Source: CAD feature listing. Evaluate the final solid. Frame: model axes, mm. A direction names the side the tool comes from. Round coordinates to 2 decimals unless told otherwise and drop trailing zeros. Loops run counter-clockwise (first coordinate to the right, second up) from the corner with the lowest first, then second, coordinate; pieces in that order, holes last.
Item 1: Pull-direction query (Y, two-part tool) for faces 1 (the cylindrical face through (266.488, 40.887, 7.465)), 2 (the flat face through (152, 25, 5)), 3 (the flat face through (161, 41, 10)); classes: released by +Y, released by -Y, zero draft, split by the parting line, or undercut.
Item 2: Section query B-B on z = 3. Return loops of the section in (x, y).
Item 3: Section query C-C on x = 206. Return loops of the section in (y, z).
Item 4: Ray query, L1, parallel to X at y = 21, z = 4; L2, parallel to Z at x = 240, y = 83; L3, parallel to Y at x = 168, z = 1. Return the intervals inside material, ascending.
Item 5: Section query D-D on x = 98.5. Return loops of the section in (y, z), then the cut area to 3 significant figures.
Item 6: Section query A-A on x = 174.5. Return loops of the section in (y, z), then the cut area to 3 significant figures.
Item 7: Access query for faces 4 (the flat face through (151, 20, 5)), 5 (the flat face through (269, 44, 2)), 6 (the flat face through (119.3, 64.4, 7.5)), 7 (the cylindrical face through (1.2, 39.8, 7.5)), 8 (the flat face through (119.291, 15.596, 7.465)). Directions: +Z, -Z, +X, -X, +Y, -Y. A direction counts if a zero-diameter tool reaches every point of the face in a straight line with its end or side. Return the directions, or none.
Item 8: First-contact query: P1, Ø2.5, axis at y = 21.5, z = 4.5, coming from the -X side; P2, Ø1, axis at y = 34.5, z = 8.5, coming from the -X side; P3, Ø5, axis at x = 160.5, z = 6, coming from the +Y side. Flat tips, straight axial feed; report the tip coordinate or a pass-through.
Autodesk Inventor part; units mm, degrees
ref_plane "YZ Plane" through (0, 0, 0) normal (1, 0, 0) x (0, 1, 0)
ref_plane "XZ Plane" through (0, 0, 0) normal (0, 1, 0) x (-1, 0, 0)
ref_plane "XY Plane" through (0, 0, 0) normal (0, 0, 1) x (1, 0, 0)
sketch "Boceto1" plane through (0, 0, 0) normal (0, 0, 1) x (1, 0, 0)
  circle A0 centre (229, 39.9983) radius 35 construction
  line L0 (269, 87.6892) -> (269, -0.002)
  line L1 (269, -0.002) -> (0, 0)
  line L2 (0, 0) -> (0, 54.8968)
  line L3 (457.9938, -0.0034) -> (457.9938, 80) construction
  line L4 (457.9938, 80) -> (-432.9938, 80) construction
  line L5 (189, -0.0014) -> (189, 79.998) construction
  line L6 (189, 79.998) -> (269, 79.998) construction
  circle A1 centre (229, 39.9983) radius 11.3 construction
  line L7 (119, 54.9966) -> (199, 54.9966) construction
  line L8 (199, 54.9966) -> (199, 25) construction
  line L9 (199, 25) -> (119, 25) construction
  line L10 (119, 25) -> (119, 54.9966) construction
  arc A2 (224.4624, 2.7754) -> (224.4624, 77.2212) centre (229, 39.9983) ccw
  arc A3 (11.1326, 51.2153) -> (11.1326, 28.7814) centre (12.5, 39.9983) ccw
  line L11 (224.4624, 77.2212) -> (11.1326, 51.2153)
  line L12 (224.4624, 2.7754) -> (11.1326, 28.7814)
  line L13 (0, 54.8968) -> (269, 87.6892)
  line L14 (119, 20) -> (184, 20)
  line L15 (119, 25) -> (119, 20)
  line L16 (184, 20) -> (184, 25)
  circle A4 centre (12.5, 39.9983) radius 3.5
  circle A5 centre (229, 39.9983) radius 3.5
  circle A6 centre (229, 39.9983) radius 30 construction
  line L17 (184, 25) -> (119, 25)
  point P0 (457.9938, 39.9983)
  point P1 (12.5, 80)
  point P2 (189, 39.9983)
  point P3 (229, 79.998)
  point P4 (199, 39.9983)
  dimension "d2" = 269
  dimension "d17" = 5
  dimension "d18" = 65
  dimension "d19" = 7
  dimension "d25" = 87.6911
  dimension "d26" = 40
  dimension "d27" = 40
  dimension "d28" = 12.5
  dimension "d29" = 39.9984
  dimension "d30" = 7
  dimension "d31" = 54.8968
extrude "Extrusión1" add sketch "Boceto1" along normal blind 5 contours L0 L1 L2 L13 | L12 A3 L11 A2
extrude "Extrusión2" add sketch "Boceto1" along normal blind 10 contours L12 A3 L11 A2
properties part number "divisores_banda"
Data:
1. face 1: split by the parting line
1. face 2: undercut
1. face 3: zero draft
2. outline: (0, 0) - (269, 0) - (269, 87.69) - (0, 54.9) - close; hole circle Ø7 at (12.5, 40); hole (119, 20) - (184, 20) - (184, 25) - (119, 25) - close; hole circle Ø7 at (229, 40)
3. outline: (0, 0) - (80.01, 0) - (80.01, 5) - (74.97, 5) - (74.97, 10) - (5.03, 10) - (5.03, 5) - (0, 5) - close
4. L1: x = 0 to 119, 184 to 269
4. L2: z = 0 to 5
4. L3: y = 0 to 20, 25 to 75.38
5. outline: (0, 0) - (66.9, 0) - (66.9, 5) - (61.87, 5) - (61.87, 10) - (18.13, 10) - (18.13, 5) - (0, 5) - close
5. area: 553 mm2
6. outline: (0, 0) - (20, 0) - (20, 10) - (8.87, 10) - (8.87, 5) - (0, 5) - close; (25, 0) - (76.17, 0) - (76.17, 5) - (71.13, 5) - (71.13, 10) - (25, 10) - close
6. area: 642 mm2
7. face 4: +Z, -Z
7. face 5: +Z, -Z, +X, +Y, -Y
7. face 6: +Z, -X, +Y
7. face 7: +Z, -X
7. face 8: +Z, -X, -Y
8. P1: stops at x = 0
8. P2: stops at x = 2.37
8. P3: stops at y = 74.74
